Part print with two shaded views. Sizes in mm from the minimum x, y, z corner. Coordinates: 2 decimals unless noted, no trailing zeros. Order: outer loops, then holes, each group sorted by start corner. A loop starts at its lowest first (then second) coordinate and runs counter-clockwise, first axis right, second up. Notation, with made-up numbers: M -40,-26.5 L 18,-26.5 A22 cw 18,-11.5 Z; hole C 9.5,12 d9. An arc over 180 degrees is marked long. Answer in a Markdown table with one row per item. Add a question column.
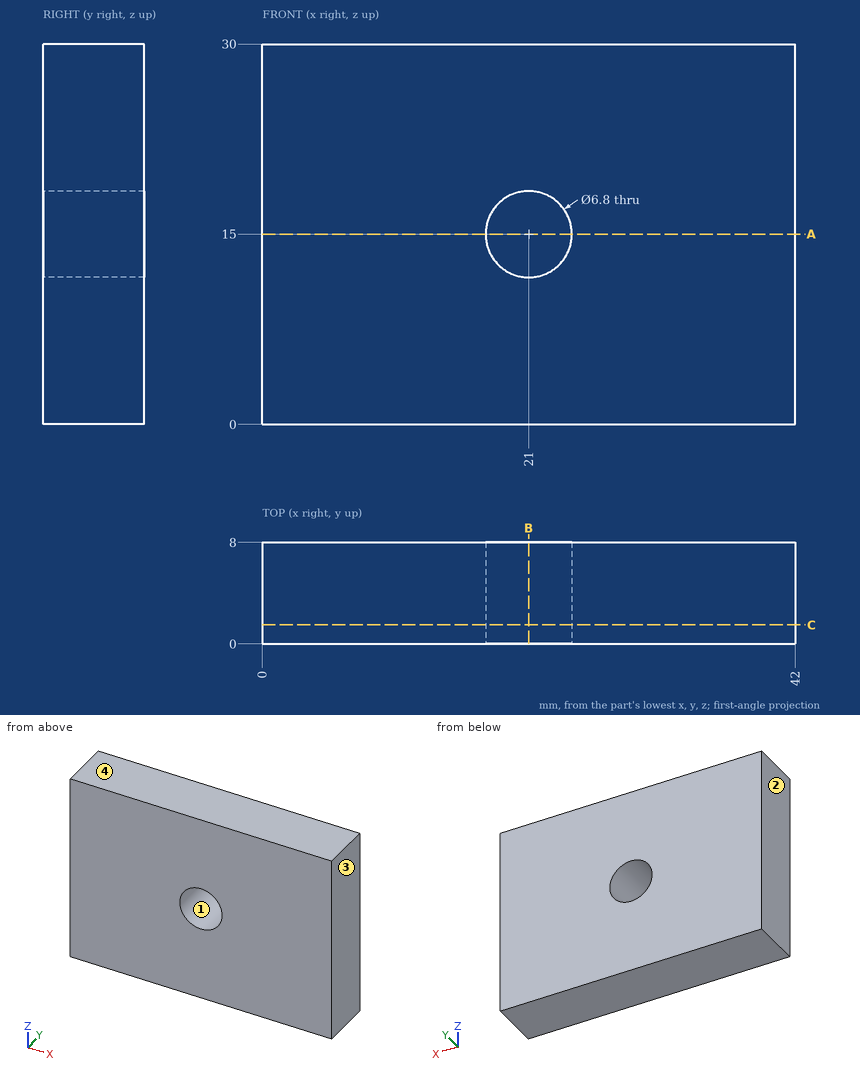
(1) Slice it at B-B (x = 21). List the corners of the cut face in (y, z).
(2) Slice it at A-A (z = 15). List the corners of the cut face in (x, y).
(3) Wall check: line 1 (Z direction, x = 21, y = 4.75); line 2 (X direction, y = 5, z = 15); line 3 (Z direction, x = 22, y = 4.75). Give the ranges that are in metal, low to high.
(4) Pull direction X, two halves, no side cores. Call the marked faces 1, 2, 3 and 4: pulls with the +X half, pulls with the -X half, needs draft (parallel to the pull), parting line crosses it, or undercut.
(5) Slice it at C-C (y = 1.5). List the corners of the cut face in (x, z).
Computed:
| question | item | result |
|---|---|---|
| 1 | outline | M 0,0 L 8,0 L 8,11.6 L 0,11.6 Z; M 0,18.4 L 8,18.4 L 8,30 L 0,30 Z |
| 2 | outline | M 0,0 L 17.6,0 L 17.6,8 L 0,8 Z; M 24.4,0 L 42,0 L 42,8 L 24.4,8 Z |
| 3 | line 1 | z = 0 to 11.6, 18.4 to 30 |
| 3 | line 2 | x = 0 to 17.6, 24.4 to 42 |
| 3 | line 3 | z = 0 to 11.75, 18.25 to 30 |
| 4 | face 1 | undercut |
| 4 | face 2 | pulls with the -X half |
| 4 | face 3 | pulls with the +X half |
| 4 | face 4 | needs draft |
| 5 | outline | M 0,0 L 42,0 L 42,30 L 0,30 Z; hole C 21,15 d6.8 |
